Part model, mm, in its own coordinate system. Face numbers are marked on the shaded views. A direction names the side the tool comes from. Round coordinates to 2 decimals unless told otherwise and drop trailing zeros. Loops run counter-clockwise (first coordinate to the right, second up) from the corner with the lowest first, then second, coordinate; pieces in that order, holes last.
1) Band-saw the part on B-B, the plane x = 28. Write the cut outline in (y, z).
2) 3-axis set-ups, long thin cutter, end or side, ignore diameter. For the marked faces 1 and 2: which of +Z, -Z, +X, -X, +Y, -Y reach the whole face in a straight line?
3) Band-saw the part on C-C, the plane y = 13.5. Write the cut outline in (x, z).
4) Band-saw the part on D-D, the plane x = 6.5. Write the cut outline in (y, z), then the cut area to 3 significant figures.
5) Probe line 1 (Y direction, x = 24.5, z = 5); line 2 (Z direction, x = 30.5, y = 8.5); line 3 (Y direction, x = 56, z = -4.5). List the from-to ranges inside material, lowest first.
6) Drop flat-ended pins along their axis: P1, Ø12, axis at y = -6, z = -16, coming from the -X side; P2, Ø1.5, axis at y = -4, z = -17.5, coming from the +X side; P3, Ø5, axis at x = 18.5, y = 2.5, coming from the -Z side; P4, Ø1, axis at y = -3, z = -30.5, coming from the +X side. Give the stop position or say it passes through.
7) Band-saw the part on A-A, the plane y = 0. Write the cut outline in (x, z), then the cut area to 3 significant figures.
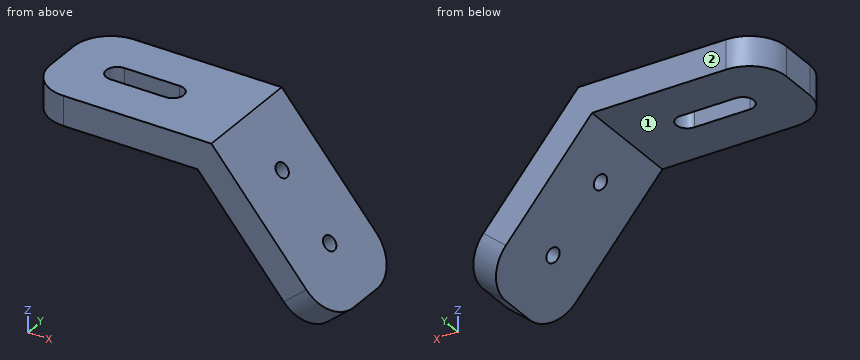
from build123d import *

# Parameters (mm, degrees)
F1_DEPTH = 15
F3_DEPTH = 43.4455230334
F5_D     = 4
F6_R     = 10


with BuildPart() as f1:
    # F0 (on Front) → F1 (new body, symmetric)
    with BuildSketch(Plane.XZ):
        Polygon((0, 8), (0, 0), (46.2695387348, 0), (76.0110249394, -35.4445230334), (82.1393804843, -30.3022221559), (50, 8), align=None)
    extrude(amount=F1_DEPTH, both=True)

    # F2 (on face) → F3 (cut, through all)
    with BuildSketch(Plane.XY.offset(8)):
        with BuildLine():
            ThreePointArc((15, 3), (12, 0), (15, -3))
            Line((15, -3), (30, -3))
            ThreePointArc((30, -3), (33, 0), (30, 3))
            Line((30, 3), (15, 3))
        make_face()
    extrude(amount=-F3_DEPTH, mode=Mode.SUBTRACT)

    # F5 (through all)
    with Locations(Plane(origin=(33.2804354537, 0, 27.9256011146), x_dir=(0, 1, 0), z_dir=(0.7660444431, 0, 0.6427876097))):
        with Locations((0, -41.0110249394), (0, -61.0110249394)):
            Hole(F5_D / 2)

    # F6
    f6_edges = [f1.edges().sort_by_distance(p)[0] for p in [
        (79.075203, -15, -32.873373),
        (79.075203, 15, -32.873373),
        (0, -15, 4),
        (0, 15, 4),
    ]]
    fillet(f6_edges, radius=F6_R)


solid = f1.part
Reported:
1. outline: (-15, 0) - (-3, 0) - (-3, 8) - (-15, 8) - close; (3, 0) - (15, 0) - (15, 8) - (3, 8) - close
2. face 1: -Z, -X, +Y, -Y
2. face 2: +Z, -Z, +X, -X, +Y
3. outline: (4.73, 0) - (46.27, 0) - (72.97, -31.82) - (79.1, -26.68) - (50, 8) - (4.73, 8) - close
4. outline: (-14.37, 0) - (14.37, 0) - (14.37, 8) - (-14.37, 8) - close
4. area: 230 mm2
5. line 1: y = -15 to -3, 3 to 15
5. line 2: z = 0 to 8
5. line 3: y = -15 to -1.24, 1.24 to 15
6. P1: stops at x = 54.66
6. P2: stops at x = 72.03
6. P3: stops at z = 0
6. P4: stops at x = 82.14
7. outline: (0, 0) - (12, 0) - (12, 8) - (0, 8) - close; (33, 0) - (46.27, 0) - (52.23, -7.1) - (58.36, -1.96) - (50, 8) - (33, 8) - close; (54.8, -10.17) - (65.08, -22.42) - (71.21, -17.28) - (60.93, -5.02) - close; (67.65, -25.49) - (76.01, -35.44) - (82.14, -30.3) - (73.78, -20.34) - close
7. area: 538 mm2
